Design review of the part built by this model. Coordinates are the model's own, in mm. Face numbers are marked on the shaded views. A direction names the side the tool comes from. Round coordinates to 2 decimals unless told otherwise and drop trailing zeros. Order: outer loops, then holes, each group sorted by start corner. A loop starts at its lowest first (then second) coordinate and runs counter-clockwise, first axis right, second up. Notation, with made-up numbers: (-36.5, 29) - (-13.5, 29) arc R14 ccw to (-13.5, 42) - close; hole circle Ø2 at (88, 38). An arc over 180 degrees is marked (long way). Write item = value, one per line.
from build123d import *

# Parameters (mm, degrees)
SKETCH1_W           = 30
SKETCH1_H           = 30
BOSS_EXTRUDE1_DEPTH = 1
SKETCH2_R           = 12.4
CUT_EXTRUDE1_DEPTH  = 22.236760582
SKETCH4_W           = 2
SKETCH4_H           = 4
SKETCH4_W_2         = 4
SKETCH4_H_2         = 2
BOSS_EXTRUDE2_DEPTH = 2
SKETCH5_W           = 4
SKETCH5_H           = 0.5
BOSS_EXTRUDE3_DEPTH = 0.8
SKETCH6_W           = 4
SKETCH6_H           = 0.5
BOSS_EXTRUDE4_DEPTH = 0.8
SKETCH7_W           = 4
SKETCH7_H           = 0.5
BOSS_EXTRUDE5_DEPTH = 0.8
SKETCH8_W           = 4
SKETCH8_H           = 0.5
BOSS_EXTRUDE6_DEPTH = 0.8
SKETCH9_W           = 2.8
SKETCH9_H           = 4
SKETCH9_W_2         = 4
SKETCH9_H_2         = 2.8
BOSS_EXTRUDE7_DEPTH = 1


with BuildPart() as part:
    # Sketch1 → Boss-Extrude1 (new body)
    with BuildSketch(Plane(origin=(0, 0, 0), x_dir=(1, 0, 0), z_dir=(0, 1, 0))):
        Rectangle(SKETCH1_W, SKETCH1_H)
    extrude(amount=BOSS_EXTRUDE1_DEPTH)

    # Sketch2 → Cut-Extrude1 (cut, through all)
    with BuildSketch(Plane(origin=(0, 1, 0), x_dir=(1, 0, 0), z_dir=(0, 1, 0))):
        with Locations(Location((0, 0, 0), (0, 0, 270))):
            Circle(SKETCH2_R)
    extrude(amount=-CUT_EXTRUDE1_DEPTH, mode=Mode.SUBTRACT)

    # Sketch4 → Boss-Extrude2 (add)
    with BuildSketch(Plane(origin=(0, 1, 0), x_dir=(1, 0, 0), z_dir=(0, 1, 0))):
        with Locations((13.7, 0)):
            Rectangle(SKETCH4_W, SKETCH4_H)
        with Locations((-13.7, 0)):
            Rectangle(SKETCH4_W, SKETCH4_H)
        with Locations((0, 13.7)):
            Rectangle(SKETCH4_W_2, SKETCH4_H_2)
        with Locations((0, -13.7)):
            Rectangle(SKETCH4_W_2, SKETCH4_H_2)
    extrude(amount=BOSS_EXTRUDE2_DEPTH)

    # Sketch5 → Boss-Extrude3 (add)
    with BuildSketch(Plane.ZY.offset(-12.7)):
        with Locations((0, 2.75)):
            Rectangle(SKETCH5_W, SKETCH5_H)
    extrude(amount=BOSS_EXTRUDE3_DEPTH)

    # Sketch6 → Boss-Extrude4 (add)
    with BuildSketch(Plane(origin=(0, 0, 12.7), x_dir=(-1, 0, 0), z_dir=(0, 0, -1))):
        with Locations((0, 2.75)):
            Rectangle(SKETCH6_W, SKETCH6_H)
    extrude(amount=BOSS_EXTRUDE4_DEPTH)

    # Sketch7 → Boss-Extrude5 (add)
    with BuildSketch(Plane(origin=(-12.7, 0, 0), x_dir=(0, 0, -1), z_dir=(1, 0, 0))):
        with Locations((0, 2.75)):
            Rectangle(SKETCH7_W, SKETCH7_H)
    extrude(amount=BOSS_EXTRUDE5_DEPTH)

    # Sketch8 → Boss-Extrude6 (add)
    with BuildSketch(Plane.XY.offset(-12.7)):
        with Locations((0, 2.75)):
            Rectangle(SKETCH8_W, SKETCH8_H)
    extrude(amount=BOSS_EXTRUDE6_DEPTH)

    # Sketch9 → Boss-Extrude7 (add)
    with BuildSketch(Plane(origin=(0, 3, 0), x_dir=(1, 0, 0), z_dir=(0, 1, 0))):
        with Locations((13.3, 0)):
            Rectangle(SKETCH9_W, SKETCH9_H)
        with Locations((-13.3, 0)):
            Rectangle(SKETCH9_W, SKETCH9_H)
        with Locations((0, -13.3)):
            Rectangle(SKETCH9_W_2, SKETCH9_H_2)
        with Locations((0, 13.3)):
            Rectangle(SKETCH9_W_2, SKETCH9_H_2)
    extrude(amount=BOSS_EXTRUDE7_DEPTH)


solid = part.part
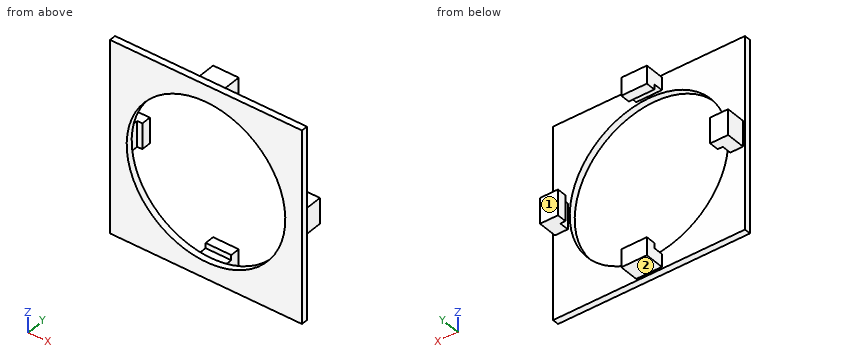
1) Clearance check with flat-ended pins moving along their axes: pin 1 Ø1.2 at (x, y) = (1, 2) entering from -Z; pin 2 Ø0.6 at (x, z) = (12, 0) entering from -Y; pin 3 Ø0.8 at (y, z) = (2, -13.5) entering from +X. State where each tip first meets the part, or that it passes through.
Findings:
pin_1 = -14.7
pin_2 = 2.5
pin_3 = 2
2) We need section C-C on y = 0.35. Write out the cut boundary in (x, z).
Findings:
outline = (-15, -15) - (15, -15) - (15, 15) - (-15, 15) - close; hole circle Ø24.8 at (0, 0)
3) We need section D-D on y = 3.25. Write out the cut boundary in (x, z), and give its area (3 significant figures).
Findings:
outline = (-14.7, -2) - (-11.9, -2) - (-11.9, 2) - (-14.7, 2) - close; (-2, -14.7) - (2, -14.7) - (2, -11.9) - (-2, -11.9) - close; (-2, 11.9) - (2, 11.9) - (2, 14.7) - (-2, 14.7) - close; (11.9, -2) - (14.7, -2) - (14.7, 2) - (11.9, 2) - close
area = 44.8 mm^2
4) We need section A-A on z = 0. Write out the cut boundary in (x, y).
Findings:
outline = (-15, 0) - (-12.4, 0) - (-12.4, 1) - (-12.7, 1) - (-12.7, 2.5) - (-11.9, 2.5) - (-11.9, 4) - (-14.7, 4) - (-14.7, 1) - (-15, 1) - close; (11.9, 2.5) - (12.7, 2.5) - (12.7, 1) - (12.4, 1) - (12.4, 0) - (15, 0) - (15, 1) - (14.7, 1) - (14.7, 4) - (11.9, 4) - close
5) We need section B-B on x = 0. Write out the cut boundary in (y, z).
Findings:
outline = (0, -15) - (1, -15) - (1, -14.7) - (4, -14.7) - (4, -11.9) - (2.5, -11.9) - (2.5, -12.7) - (1, -12.7) - (1, -12.4) - (0, -12.4) - close; (0, 12.4) - (1, 12.4) - (1, 12.7) - (2.5, 12.7) - (2.5, 11.9) - (4, 11.9) - (4, 14.7) - (1, 14.7) - (1, 15) - (0, 15) - close
6) To check wall thickness, follow L1, parallel to X at y = 0.5, z = 0; L2, parallel to Z at x = 0.5, y = 1.55; L3, parallel to X at y = 3.85, z = -1.5. State the ranges of each line that lie inside material, in increasing order. Write a range as from..to.
Findings:
L1 = -15..-12.4, 12.4..15
L2 = -14.7..-12.7, 12.7..14.7
L3 = -14.7..-11.9, 11.9..14.7
7) For the marked faces 1 and 2, list the 3-axis set-ups (+Z, -Z, +X, -X, +Y, -Y) from which the entire face can be reached by the end or side of a thin tool; tool diameter is ignored.
Findings:
face_1 = +Z, -Z, +X, -X, +Y
face_2 = -Z, +X, -X, +Y
